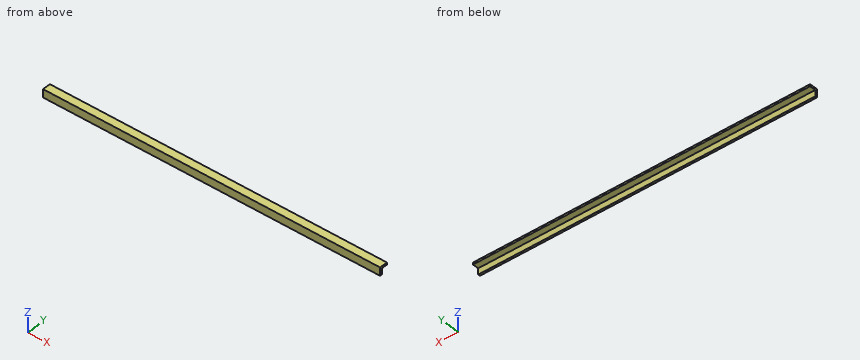
from build123d import *

# Parameters (mm, degrees)
BOSS_EXTRUDE1_DEPTH      = 533.4
BOSS_EXTRUDE1_DEPTH_BACK = 533.4


with BuildPart() as part:
    # Sketch1 → Boss-Extrude1 (new body, two sides)
    with BuildSketch(Plane(origin=(0, 0, 0), x_dir=(0, 0, -1), z_dir=(1, 0, 0))) as boss_extrude1_sk:
        Polygon((25.4, 6.35), (25.4, 0), (0, 0), (0, 25.4), (6.35, 25.4), (6.35, 6.35), align=None)
    extrude(amount=BOSS_EXTRUDE1_DEPTH)
    extrude(boss_extrude1_sk.sketch, amount=-BOSS_EXTRUDE1_DEPTH_BACK)


solid = part.part
Could you check a few things on this model? Use its own coordinates, in mm. Give positions to 0.01 mm unless a question says otherwise; leave off trailing zeros. Write each loop counter-clockwise with the first axis right and the second up, starting at its lowest first coordinate (ties: lowest second). Pieces come first, ordered by that corner, then holes. Notation, with made-up numbers: (20.25, -31.75) - (69.25, -31.75) arc R28 ccw to (69.25, -2.75) - close; hole circle Ø5 at (-28, 44). An arc over 180 degrees is marked (long way). Use CSV: the item, a comma, the result in double quotes. Start each with the question number.
Item 1: I want a section at C-C, the plane y = 10.5. Please give me the cut outline in (x, z).
Item 2: I want a section at A-A, the plane x = 263.5. Please give me the cut outline in (y, z), then the cut area to 3 significant figures.
Item 3: I want a section at B-B, the plane z = -19. Please give me the cut outline in (x, y), then the cut area to 3 significant figures.
Item 4: I'm going to push flat-ended pins straight in: pin 1 (2 mm diameter, centred on x = -273, y = 13.5, fed in from -Z); pin 2 (15 mm diameter, centred on x = 84, z = -15, fed in from +Y). Where does each tip first touch, or does it pass through?
Item 5: If I drill on line 1 along Y through (x, z) = (-387, -11); line 2 along Z through (x, y) = (-115, 18.5), over which ranges is the centre line in solid material (lowest first)?
Findings:
1,outline,"(-533.4, -6.35) - (533.4, -6.35) - (533.4, 0) - (-533.4, 0) - close"
2,outline,"(0, -25.4) - (6.35, -25.4) - (6.35, -6.35) - (25.4, -6.35) - (25.4, 0) - (0, 0) - close"
2,area,"282 mm2"
3,outline,"(-533.4, 0) - (533.4, 0) - (533.4, 6.35) - (-533.4, 6.35) - close"
3,area,"6,770 mm2"
4,pin 1,"stops at z = -6.35"
4,pin 2,"stops at y = 6.35"
5,line 1,"y = 0 to 6.35"
5,line 2,"z = -6.35 to 0"
